Design review of the part built by this model. Coordinates are the model's own, in mm. A direction names the side the tool comes from. Give positions to 0.01 mm unless a question says otherwise; leave off trailing zeros. Loops run counter-clockwise (first coordinate to the right, second up) from the corner with the lowest first, then second, coordinate; pieces in that order, holes last. Notation, with made-up numbers: M -35,48 L 9,48 A20 ccw 9,80 Z; hole C 33,-28 d4. An arc over 180 degrees is marked long. Answer as CSV lines item,"result".
Autodesk Inventor part; units mm, degrees
ref_plane "YZ Plane" through (0, 0, 0) normal (1, 0, 0) x (0, 1, 0)
ref_plane "XZ Plane" through (0, 0, 0) normal (0, 1, 0) x (-1, 0, 0)
ref_plane "XY Plane" through (0, 0, 0) normal (0, 0, 1) x (1, 0, 0)
sketch "Skizze1" plane through (0, 0, 0) normal (0, 0, 1) x (1, 0, 0)
  line L0 (12.8939, 18.6723) -> (2.8939, 18.6723)
  line L1 (2.8939, 18.6723) -> (2.8939, 15.6723)
  line L2 (2.8939, 15.6723) -> (12.8939, 15.6723)
  line L3 (12.8939, 15.6723) -> (12.8939, 18.6723)
  line L4 (12.8939, 9.0723) -> (2.8939, 9.0723)
  line L5 (2.8939, 9.0723) -> (2.8939, 6.0723)
  line L6 (2.8939, 6.0723) -> (12.8939, 6.0723)
  line L7 (12.8939, 6.0723) -> (12.8939, 9.0723)
  line L8 (12.8939, 15.6723) -> (12.8939, 12.3723) construction
  line L9 (12.8939, 12.3723) -> (12.8939, 9.0723) construction
  point P0 (0, 0)
  point P1 (7.8939, 9.0723)
  dimension "d0" = 10
  dimension "d1" = 3
  dimension "d2" = 3
  dimension "d3" = 6.6
extrude "Extrusion1" add sketch "Skizze1" along normal blind 20
fillet "Rundung1" radius 3 4 edges at (12.8939, 7.5723, 20) (12.8939, 17.1723, 20) (2.8939, 17.1723, 20) (2.8939, 7.5723, 20)
sketch "Skizze2" plane through (2.8939, 6.0723, 0) normal (0, -1, 0) x (1, 0, 0)
  circle A0 centre (5, 15) radius 5 construction
  line L0 (10, 0) -> (10, 17) construction
  line L1 (0, 0) -> (0, 17) construction
  line L2 (3, 20) -> (7, 20) construction
  point P0 (-2.8939, 0)
hole "Bohrung1" at (7.8939, 6.0723, 15) direction (0, 1, 0) diameter 3.242 end through all countersink diameter 9 countersink angle 90
sketch "Skizze3" plane through (2.8939, 15.6723, 0) normal (0, -1, 0) x (1, 0, 0)
  line L0 (0, 0) -> (10, 0)
  line L1 (10, 0) -> (10, 2)
  line L2 (10, 0) -> (10, 17)
  line L3 (10, 2) -> (0, 2)
  line L4 (0, 0) -> (0, 17)
  point P0 (-2.8939, 0)
  dimension "d15" = 2
extrude "Extrusion2" add sketch "Skizze3" along normal through all
sketch "Skizze4" plane through (2.8939, 15.6723, 2) normal (0, 0, 1) x (1, 0, 0)
  line L0 (10, -3.3) -> (10, 0) construction
  line L1 (10, -3.3) -> (10, -6.6) construction
  line L2 (0, -3.3) -> (0, -6.6) construction
  line L3 (0, 0) -> (0, -3.3) construction
  line L4 (7, 3) -> (3, 3) construction
  line L5 (0, 3) -> (0, 0) construction
  line L6 (-4, -3.3) -> (5, -3.3) construction
  line L7 (-4, -3.3) -> (5, -3.3) construction
  line L8 (-4, -3.3) -> (5, -3.3) construction
  line L9 (2.5, -3.3) -> (5, -3.3) construction
  line L10 (5, -3.3) -> (7.5, -3.3) construction
  point P0 (-2.8939, -15.6723)
  dimension "d34" = 5
  dimension "d35" = 9
  dimension "d36" = 6.3
  dimension "d37" = 5
  dimension "d38" = 9
  dimension "d40" = 9
  dimension "d41" = 0
hole "Bohrung2" at (10.3939, 12.3723, 2) at (5.3939, 12.3723, 2) direction (0, 0, -1) diameter 2 end through all countersink diameter 5 countersink angle 90
sketch "Skizze5" plane through (2.8939, 6.0723, 0) normal (0, -1, 0) x (1, 0, 0)
  circle A0 centre (5, 15) radius 4.5
  point P0 (-2.8939, 0)
hole "Bohrung3" at (7.8939, 6.0723, 15) direction (0, 1, 0) diameter 4 depth 3
properties part number "HalterUmlenkrolleOVR" material "PC/ABS-Kunststoff, 3DDruck, PLA"
1. For P1, Ø3.5, axis at x = 5.5, y = 11, coming from the +Z side; P2, Ø2, axis at x = 7, z = 13.5, coming from the -Y side, all flat-tipped, find the tip position at first contact; note any pin that passes through.
Answer block:
P1,"z = 2"
P2,"y = 7.83"
2. We need section A-A, the plane z = 7.5. Write out the cut boundary in (x, y).
Answer block:
outline,"M 2.89,6.07 L 12.89,6.07 L 12.89,9.07 L 2.89,9.07 Z; M 2.89,15.67 L 12.89,15.67 L 12.89,18.67 L 2.89,18.67 Z"
3. For faces 1 (the flat face through (8, 18.672, 10)), 2 (the flat face through (8, 9.072, 11)), 3 (the cylindrical face through (9.67, 8.83, 14.08)), list the 3-axis set-ups (+Z, -Z, +X, -X, +Y, -Y) from which the entire face can be reached by the end or side of a thin tool; tool diameter is ignored.
Answer block:
face 1,"+Z, -Z, +X, -X, +Y"
face 2,"+Z, +X, -X"
face 3,"-Y"
4. We need section C-C, the plane y = 18. Write out the cut boundary in (x, z), plus the area to 3 significant figures.
Answer block:
outline,"M 2.89,0 L 12.89,0 L 12.89,17 A3 ccw 9.89,20 L 5.89,20 A3 ccw 2.89,17 Z; hole C 7.89,15 d3.24"
area,"188 mm²"
5. The part is to be moulded in two halves that separate along X. For faces 4 (the flat face through (8, 15.672, 11)), 5 (the cylindrical face through (11.37, 12.59, 0.25)), 6 (the cylindrical face through (3.796, 7.551, 19.145)), say which applies: pulls with the +X half, pulls with the -X half, needs draft (parallel to the pull), parting line crosses it, or undercut.
Answer block:
face 4,"needs draft"
face 5,"undercut"
face 6,"pulls with the -X half"
6. We need section B-B, the plane z = 15. Write out the cut boundary in (x, y).
Answer block:
outline,"M 2.89,6.07 L 3.39,6.07 L 5.89,8.57 L 5.89,9.07 L 2.89,9.07 Z; M 2.89,15.67 L 6.27,15.67 L 6.27,18.67 L 2.89,18.67 Z; M 9.51,15.67 L 12.89,15.67 L 12.89,18.67 L 9.51,18.67 Z; M 9.89,8.57 L 12.39,6.07 L 12.89,6.07 L 12.89,9.07 L 9.89,9.07 Z"
7. To check wall thickness, follow L1, parallel to X at y = 8.9, z = 15; L2, parallel to Y at x = 11.5, z = 7.5; L3, parallel to Y at x = 4.75, z = 17.75. State the ranges of each line that lie inside material, in increasing order. Write a range as [from, to].
Answer block:
L1,"[2.89, 5.89], [9.89, 12.89]"
L2,"[6.07, 9.07], [15.67, 18.67]"
L3,"[6.4, 9.07], [15.67, 18.67]"
8. We need section D-D, the plane y = 15.25. Write out the cut boundary in (x, z).
Answer block:
outline,"M 2.89,0 L 12.89,0 L 12.89,2 L 2.89,2 Z"
